Read the model definition and answer for the solid it produces. Units are mm, in the model's axes. A direction names the side the tool comes from. Coordinates: 2 decimals unless noted, no trailing zeros. Order: outer loops, then holes, each group sorted by start corner. A loop starts at its lowest first (then second) coordinate and runs counter-clockwise, first axis right, second up.
from build123d import *

# Parameters (mm, degrees)
SKETCH2_W               = 6.1
SKETCH2_H               = 8
CUT_EXTRUDE1_DEPTH      = 22
CUT_EXTRUDE1_DEPTH_BACK = 22
SKETCH3_R               = 2.325
CUT_EXTRUDE2_DEPTH      = 10


with BuildPart() as part:
    # Sketch1 → Revolve1 (revolve)
    with BuildSketch(Plane(origin=(0, 0, 0), x_dir=(0, 0, -1), z_dir=(1, 0, 0))):
        Polygon((14.5, 6), (-14.5, 6), (-14.5, 8), (-17.5, 8), (-17.5, 21), (-9.5, 21), (-9.5, 11), (17.5, 11), (17.5, 8), (14.5, 8), align=None)
    revolve(axis=Axis((0, 0, 27), (0, 0, -1)))

    # Sketch2 → Cut-Extrude1 (cut, two sides)
    with BuildSketch(Plane(origin=(0, 0, 0), x_dir=(1, 0, 0), z_dir=(0, 1, 0))) as cut_extrude1_sk:
        with Locations((-17.95, -13.5)):
            Rectangle(SKETCH2_W, SKETCH2_H)
        with Locations((17.95, -13.5)):
            Rectangle(SKETCH2_W, SKETCH2_H)
    extrude(amount=CUT_EXTRUDE1_DEPTH, mode=Mode.SUBTRACT)
    extrude(cut_extrude1_sk.sketch, amount=-CUT_EXTRUDE1_DEPTH_BACK, mode=Mode.SUBTRACT)

    # Sketch3 → Cut-Extrude2 (cut)
    with BuildSketch(Plane.XY.offset(17.5)):
        with Locations((0, 16)):
            Circle(SKETCH3_R)
        with Locations((11.313708499, 11.313708499)):
            Circle(SKETCH3_R)
        with Locations((11.313708499, -11.313708499)):
            Circle(SKETCH3_R)
        with Locations((0, -16)):
            Circle(SKETCH3_R)
        with Locations((-11.313708499, -11.313708499)):
            Circle(SKETCH3_R)
        with Locations((-11.313708499, 11.313708499)):
            Circle(SKETCH3_R)
    extrude(amount=-CUT_EXTRUDE2_DEPTH, mode=Mode.SUBTRACT)


solid = part.part
Q1. The part is cut by section A-A, the plane y = 0. Determine the outline of the cut face in (x, z), then the cut area to 3 significant figures.
Q2. Which of the six approach directions +Z, -Z, +X, -X, +Y, -Y give full straight-line access (tool end or side, diameter ignored) to faces 1 (the cylindrical face through (0, 21, 13)), 2 (the flat face through (6, 2, 14.5)), 3 (the cylindrical face through (-7.81, -1.73, -15.98))?
Q3. Determine the mould class of faces 4 (the flat face through (7, 9, 9.5)), 5 (the cylindrical face through (-10.74, -2.38, -4.19)), 6 (the cylindrical face through (-0.303, 18.305, 13.556)) for opening direction X: +X half, -X half, draft (parallel to the pull), parting line (faces both ways), or undercut.
Q4. The part is cut by section D-D, the plane y = 10.5. Determine the outline of the cut face in (x, z), then the cut area to 3 significant figures.
Q5. The part is cut by section B-B, the plane x = 0. Determine the outline of the cut face in (y, z) (3 decimals), then the cut area to 3 significant figures.
Q6. Straight lines are drawn through the part: L1, parallel to X at y = 11.5, z = 14.5; L2, parallel to X at y = 0, z = 6.5; L3, parallel to X at y = -12, z = 15. For each, find the intervals that lie inside material, in ascending order.
Q7. Each of these flat-tipped pins is pushed along its axis until it touches: P1, Ø5.5, axis at x = 0, y = -16, coming from the +Z side; P2, Ø3.5, axis at x = 11.31, y = 11.31, coming from the +Z side; P3, Ø1.5, axis at x = 10, z = 10.5, coming from the +Y side; P4, Ø14, axis at x = 0, y = 0, coming from the -Z side. Where does it stop, or does it pass through?
Q8. The part is cut by section C-C, the plane x = 4.75. Determine the outline of the cut face in (y, z), then the cut area to 3 significant figures.
Computed values:
1. outline: (-14.9, 9.5) - (-11, 9.5) - (-11, -17.5) - (-8, -17.5) - (-8, -14.5) - (-6, -14.5) - (-6, 14.5) - (-8, 14.5) - (-8, 17.5) - (-14.9, 17.5) - close; (6, -14.5) - (8, -14.5) - (8, -17.5) - (11, -17.5) - (11, 9.5) - (14.9, 9.5) - (14.9, 17.5) - (8, 17.5) - (8, 14.5) - (6, 14.5) - close
1. area: 388 mm2
2. face 1: +Z, -Z, +Y
2. face 2: +Z
2. face 3: -Z
3. face 4: draft
3. face 5: parting line
3. face 6: undercut
4. outline: (-14.9, 9.5) - (-13.49, 9.5) - (-13.49, 17.5) - (-14.9, 17.5) - close; (-9.14, 9.5) - (-3.28, 9.5) - (-3.28, -17.5) - (3.28, -17.5) - (3.28, 9.5) - (9.14, 9.5) - (9.14, 17.5) - (-9.14, 17.5) - close; (13.49, 9.5) - (14.9, 9.5) - (14.9, 17.5) - (13.49, 17.5) - close
4. area: 346 mm2
5. outline: (-21, 9.5) - (-18.325, 9.5) - (-18.325, 17.5) - (-21, 17.5) - close; (-13.675, 9.5) - (-11, 9.5) - (-11, -17.5) - (-8, -17.5) - (-8, -14.5) - (-6, -14.5) - (-6, 14.5) - (-8, 14.5) - (-8, 17.5) - (-13.675, 17.5) - close; (6, -14.5) - (8, -14.5) - (8, -17.5) - (11, -17.5) - (11, 9.5) - (13.675, 9.5) - (13.675, 17.5) - (8, 17.5) - (8, 14.5) - (6, 14.5) - close; (18.325, 9.5) - (21, 9.5) - (21, 17.5) - (18.325, 17.5) - close
5. area: 412 mm2
6. L1: x = -14.9 to -13.63, -9 to 9, 13.63 to 14.9
6. L2: x = -11 to -6, 6 to 11
6. L3: x = -14.9 to -13.54, -9.09 to 9.09, 13.54 to 14.9
7. P1: stops at z = 17.5
7. P2: passes through
7. P3: stops at y = 18.85
7. P4: stops at z = -14.5
8. outline: (-20.46, 9.5) - (-9.92, 9.5) - (-9.92, -17.5) - (-6.44, -17.5) - (-6.44, -14.5) - (-3.67, -14.5) - (-3.67, 14.5) - (-6.44, 14.5) - (-6.44, 17.5) - (-20.46, 17.5) - close; (3.67, -14.5) - (6.44, -14.5) - (6.44, -17.5) - (9.92, -17.5) - (9.92, 9.5) - (20.46, 9.5) - (20.46, 17.5) - (6.44, 17.5) - (6.44, 14.5) - (3.67, 14.5) - close
8. area: 573 mm2
